```python
from build123d import *

# Parameters (mm, degrees)
SKETCH_1_R      = 1.5
SKETCH_1_R_2    = 1.55
SKETCH_1_W      = 10
SKETCH_1_H      = 6.1
SKETCH_1_W_2    = 15.1
SKETCH_1_W_3    = 6.1
SKETCH_1_H_2    = 15
SKETCH_1_W_4    = 6
SKETCH_1_H_3    = 10
EXTRUDE_1_DEPTH = 6


with BuildPart() as part:
    # Эскиз1 → Бобышка-Вытянуть1 (new body)
    with BuildSketch(Plane.XY):
        with BuildLine():
            Line((-29, 222.1), (-29, 181.1))
            ThreePointArc((-29, 181.1), (-27.828427125, 178.271572875), (-25, 177.1))
            Line((-25, 177.1), (-14, 177.1))
            ThreePointArc((-14, 177.1), (-6.928932188, 174.171067812), (-4, 167.1))
            Line((-4, 167.1), (-4, -167.1))
            ThreePointArc((-4, -167.1), (-6.928932188, -174.171067812), (-14, -177.1))
            Line((-14, -177.1), (-25, -177.1))
            ThreePointArc((-25, -177.1), (-27.828427125, -178.271572875), (-29, -181.1))
            Line((-29, -181.1), (-29, -222.1))
            ThreePointArc((-29, -222.1), (-28.121320344, -224.221320344), (-26, -225.1))
            Line((-26, -225.1), (25, -225.1))
            ThreePointArc((25, -225.1), (27.828427125, -223.928427125), (29, -221.1))
            Line((29, -221.1), (29, 221.1))
            ThreePointArc((29, 221.1), (27.828427125, 223.928427125), (25, 225.1))
            Line((25, 225.1), (-26, 225.1))
            ThreePointArc((-26, 225.1), (-28.121320344, 224.221320344), (-29, 222.1))
        make_face()
        with Locations((22, 171.1)):
            Circle(SKETCH_1_R, mode=Mode.SUBTRACT)
        with Locations((13, 186.1)):
            Circle(SKETCH_1_R, mode=Mode.SUBTRACT)
        with Locations((-1, 220.1)):
            Circle(SKETCH_1_R, mode=Mode.SUBTRACT)
        with Locations((-15, 186.1)):
            Circle(SKETCH_1_R, mode=Mode.SUBTRACT)
        with Locations((22, 103.1)):
            Circle(SKETCH_1_R_2, mode=Mode.SUBTRACT)
        with Locations((22, -171.1)):
            Circle(SKETCH_1_R, mode=Mode.SUBTRACT)
        with Locations((13, -186.1)):
            Circle(SKETCH_1_R, mode=Mode.SUBTRACT)
        with Locations((-1, -220.1)):
            Circle(SKETCH_1_R, mode=Mode.SUBTRACT)
        with Locations((-15, -186.1)):
            Circle(SKETCH_1_R, mode=Mode.SUBTRACT)
        with Locations((22, -103.1)):
            Circle(SKETCH_1_R_2, mode=Mode.SUBTRACT)
        with Locations((-10, 220.05)):
            Rectangle(SKETCH_1_W, SKETCH_1_H, mode=Mode.SUBTRACT)
        with Locations((-1, 186.05)):
            Rectangle(SKETCH_1_W_2, SKETCH_1_H, mode=Mode.SUBTRACT)
        with Locations((8, 220.05)):
            Rectangle(SKETCH_1_W, SKETCH_1_H, mode=Mode.SUBTRACT)
        with Locations((-24, 206.1)):
            Rectangle(SKETCH_1_W_3, SKETCH_1_H_2, mode=Mode.SUBTRACT)
        with Locations((22, 206.1)):
            Rectangle(SKETCH_1_W_3, SKETCH_1_H_2, mode=Mode.SUBTRACT)
        with Locations((22, 52.1)):
            Rectangle(SKETCH_1_W_4, SKETCH_1_H_3, mode=Mode.SUBTRACT)
        with Locations((22, 154.1)):
            Rectangle(SKETCH_1_W_4, SKETCH_1_H_3, mode=Mode.SUBTRACT)
        with Locations((-10, -220.05)):
            Rectangle(SKETCH_1_W, SKETCH_1_H, mode=Mode.SUBTRACT)
        with Locations((-1, -186.05)):
            Rectangle(SKETCH_1_W_2, SKETCH_1_H, mode=Mode.SUBTRACT)
        with Locations((8, -220.05)):
            Rectangle(SKETCH_1_W, SKETCH_1_H, mode=Mode.SUBTRACT)
        with Locations((-24, -206.1)):
            Rectangle(SKETCH_1_W_3, SKETCH_1_H_2, mode=Mode.SUBTRACT)
        with Locations((22, -206.1)):
            Rectangle(SKETCH_1_W_3, SKETCH_1_H_2, mode=Mode.SUBTRACT)
        with Locations((22, -52.1)):
            Rectangle(SKETCH_1_W_4, SKETCH_1_H_3, mode=Mode.SUBTRACT)
        with Locations((22, -154.1)):
            Rectangle(SKETCH_1_W_4, SKETCH_1_H_3, mode=Mode.SUBTRACT)
    extrude(amount=EXTRUDE_1_DEPTH)


solid = part.part
```
The listing builds one solid part. Answer for the finished solid, in the listing's coordinates (mm). Coordinates: 2 decimals unless noted, no trailing zeros. Loops run counter-clockwise (first coordinate to the right, second up) from the corner with the lowest first, then second, coordinate; pieces in that order, holes last. Notation, with made-up numbers: M 23.5,18.25 L 29.5,18.25 A33 ccw 29.5,57.25 Z; hole C 46,26.25 d4. An arc over 180 degrees is marked long. Answer as a JSON object with one key per item and string values. Group by question number.
Item 1: Section A-A (z = 2.05) is taken. Give the number of separate pieces and of enclosed holes in the cut face, and give its area (3 significant figures).
Item 2: Consider L1, parallel to Y at x = -1, z = 4; L2, parallel to Y at x = -21.5, z = 2.5; L3, parallel to Y at x = 9, z = 4.9. Determine where each line is inside the solid, lowest interval first.
Item 3: This flat-tipped pin is pushed along its axis until it touches: P1, Ø1.8, axis at y = -50, z = 3.5, coming from the -X side. Where does it stop, or does it pass through?
Item 4: Determine the mould class of faces 1 (the face through (-7.01, 174.25, 2.96)), 2 (the face through (-6.85, -174.09, 2.96)), 3 (the face through (6, 3, 0)) for opening direction Y: +Y half, -Y half, draft (parallel to the pull), parting line (faces both ways), or undercut.
Item 5: Section B-B (y = -5.5) is taken. Write down the section's boundary in (x, z).
Solved:
{
 "1": {"separate pieces": "1", "enclosed holes": "24", "area": "16,200 mm2"},
 "2": {"L1": "y = -225.1 to -221.6, -218.6 to -189.1, -183 to 183, 189.1 to 218.6, 221.6 to 225.1", "L2": "y = -225.1 to -213.6, -198.6 to -177.1, 177.1 to 198.6, 213.6 to 225.1", "L3": "y = -225.1 to -223.1, -217 to 217, 223.1 to 225.1"},
 "3": {"P1": "stops at x = -4"},
 "4": {"face 1": "undercut", "face 2": "undercut", "face 3": "draft"},
 "5": {"outline": "M -4,0 L 29,0 L 29,6 L -4,6 Z"}
}
